CAD build for the part. Positions are in the model's coordinates, mm. A direction names the side the tool comes from. Coordinates: 2 decimals unless noted, no trailing zeros. Loops run counter-clockwise (first coordinate to the right, second up) from the corner with the lowest first, then second, coordinate; pieces in that order, holes last. Notation, with made-up numbers: (70, -12) - (95, -12) arc R21 ccw to (95, -4) - close; hole circle Ø3 at (19, 24). An arc over 180 degrees is marked (long way). Put each result on its own line as item: value.
```python
from build123d import *

# Parameters (mm, degrees)
BOSS_EXTRUDE1_DEPTH = 40
SKETCH2_R           = 6
CUT_EXTRUDE1_DEPTH  = 395
SKETCH3_R           = 5
CUT_EXTRUDE2_DEPTH  = 50


with BuildPart() as part:
    # Sketch1 → Boss-Extrude1 (new body)
    with BuildSketch(Plane(origin=(0, 0, 0), x_dir=(1, 0, 0), z_dir=(0, 1, 0))):
        Polygon((0, 170), (180, 170), (180, 130), (40, 130), (40, -130), (180, -130), (180, -170), (0, -170), align=None)
    extrude(amount=BOSS_EXTRUDE1_DEPTH)

    # Sketch2 → Cut-Extrude1 (cut)
    with BuildSketch(Plane.XY.offset(170)):
        with Locations((110, 20)):
            Circle(SKETCH2_R)
    extrude(amount=-CUT_EXTRUDE1_DEPTH, mode=Mode.SUBTRACT)

    # Sketch3 → Cut-Extrude2 (cut)
    with BuildSketch(Plane(origin=(180, 0, 0), x_dir=(0, 0, -1), z_dir=(1, 0, 0))):
        with Locations((-150, 20)):
            Circle(SKETCH3_R)
        with Locations(Location((150, 20, 0), (0, 0, 180))):
            Circle(SKETCH3_R)
    extrude(amount=-CUT_EXTRUDE2_DEPTH, mode=Mode.SUBTRACT)


solid = part.part
```
Q1. Mould opens along X. For faces 4 (the cylindrical face through (104, 20, 150)), 5 (the flat face through (180, 15, -146)), 6 (the flat face through (31, 40, -2)) say: +X half, -X half, draft (parallel to the pull), parting line (faces both ways), or undercut.
Determined:
face 4: undercut
face 5: +X half
face 6: draft
Q2. Pin check, flat tips, straight feed: pin 1 Ø6 at (y, z) = (11.5, 20) entering from -X; pin 2 Ø7 at (x, y) = (110, 20) entering from -Z. Stop position of each tip, or through.
Determined:
pin 1: x = 0
pin 2: through
Q3. Slice it at B-B, the plane x = 110. Give the cut face in (y, z), then the cut area to 3 significant figures.
Determined:
outline: (0, -170) - (14, -170) - (14, -130) - (0, -130) - close; (0, 130) - (14, 130) - (14, 170) - (0, 170) - close; (26, -170) - (40, -170) - (40, -130) - (26, -130) - close; (26, 130) - (40, 130) - (40, 170) - (26, 170) - close
area: 2,240 mm2
Q4. Tool access for faces 1 (the flat face through (91, 20, 170)), 2 (the flat face through (109, 11, 130)), 3 (the flat face through (130, 20, -150)): list every direction of +Z, -Z, +X, -X, +Y, -Y with a clear straight run to the whole face (end or side of a thin tool).
Determined:
face 1: +Z, +X, -X, +Y, -Y
face 2: +X, +Y, -Y
face 3: +X
Q5. Slice it at D-D, the plane y = 4.5. Give the cut face in (x, z).
Determined:
outline: (0, -170) - (180, -170) - (180, -130) - (40, -130) - (40, 130) - (180, 130) - (180, 170) - (0, 170) - close
Q6. Slice it at A-A, the plane x = 135.5. Give the cut face in (y, z).
Determined:
outline: (0, -170) - (40, -170) - (40, -130) - (0, -130) - close; (0, 130) - (40, 130) - (40, 170) - (0, 170) - close; hole circle Ø10 at (20, -150); hole circle Ø10 at (20, 150)
Q7. Slice it at C-C, the plane z = -150. Give the cut face in (x, y), then the cut area to 3 significant figures.
Determined:
outline: (0, 0) - (180, 0) - (180, 15) - (130, 15) - (130, 25) - (180, 25) - (180, 40) - (0, 40) - close; hole circle Ø12 at (110, 20)
area: 6,590 mm2
Q8. Wall check: L1, parallel to Y at x = 110, z = 141; L2, parallel to Z at x = 104, y = 9.5; L3, parallel to X at y = 8, z = 1. Give the ranges that are in metal, low to high. Write a range as from..to.
Determined:
L1: 0..14, 26..40
L2: -170..-130, 130..170
L3: 0..40
